```python
from build123d import *

# Parameters (mm, degrees)
ESQUISSE1_W             = 15
ESQUISSE1_H             = 11
BOSS_EXTRU_1_DEPTH      = 7.5
ESQUISSE2_R             = 1.5
ENL_V_MAT_EXTRU_1_DEPTH = 12.947803145
CONG_1_R                = 2
CONG_2_R                = 0.5


with BuildPart() as part:
    # Esquisse1 → Boss.-Extru.1 (new body)
    with BuildSketch(Plane.XY):
        Rectangle(ESQUISSE1_W, ESQUISSE1_H)
    extrude(amount=BOSS_EXTRU_1_DEPTH)

    # Esquisse2 → Enlèv. mat.-Extru.1 (cut, through all)
    with BuildSketch(Plane.XY.offset(7.5)):
        with Locations((0, 2)):
            Circle(ESQUISSE2_R)
    extrude(amount=-ENL_V_MAT_EXTRU_1_DEPTH, mode=Mode.SUBTRACT)

    # Congé1
    cong_1_edges = [part.edges().sort_by_distance(p)[0] for p in [
        (-7.5, 5.5, 3.75),
        (7.5, 5.5, 3.75),
    ]]
    fillet(cong_1_edges, radius=CONG_1_R)

    # Congé2
    cong_2_edges = [part.edges().sort_by_distance(p)[0] for p in [
        (7.5, -5.5, 3.75),
        (-7.5, -5.5, 3.75),
    ]]
    fillet(cong_2_edges, radius=CONG_2_R)


solid = part.part
```
Work out the finished part from the listing and answer in its coordinate system (mm). Give positions to 0.01 mm unless a question says otherwise; leave off trailing zeros. Write each loop counter-clockwise with the first axis right and the second up, starting at its lowest first coordinate (ties: lowest second). Pieces come first, ordered by that corner, then holes. Notation, with made-up numbers: (-24, 82) -> (10, 82) arc R24 cw to (10, 118) -> close; hole circle Ø5 at (65.25, 53). An arc over 180 degrees is marked (long way). Write item = value, one per line.
Q1. Section A-A on y = 2 is taken. Determine the outline of the cut face in (x, z).
Computed values:
outline = (-7.5, 0) -> (-1.5, 0) -> (-1.5, 7.5) -> (-7.5, 7.5) -> close; (1.5, 0) -> (7.5, 0) -> (7.5, 7.5) -> (1.5, 7.5) -> close
Q2. Consider line 1 along Y through (x, z) = (0, 3.25); line 2 along X through (y, z) = (2.5, 5); line 3 along X through (y, z) = (1.25, 4.75). Determine where each line is inside the solid, lowest interval first.
Computed values:
line_1 = -5.5 to 0.5, 3.5 to 5.5
line_2 = -7.5 to -1.41, 1.41 to 7.5
line_3 = -7.5 to -1.3, 1.3 to 7.5
Q3. Section B-B on x = 0 is taken. Determine the outline of the cut face in (y, z).
Computed values:
outline = (-5.5, 0) -> (0.5, 0) -> (0.5, 7.5) -> (-5.5, 7.5) -> close; (3.5, 0) -> (5.5, 0) -> (5.5, 7.5) -> (3.5, 7.5) -> close
Q4. Section C-C on z = 1.5 is taken. Determine the outline of the cut face in (x, y), and give its area (3 significant figures).
Computed values:
outline = (-7.5, -5) arc R0.5 ccw to (-7, -5.5) -> (7, -5.5) arc R0.5 ccw to (7.5, -5) -> (7.5, 3.5) arc R2 ccw to (5.5, 5.5) -> (-5.5, 5.5) arc R2 ccw to (-7.5, 3.5) -> close; hole circle Ø3 at (0, 2)
area = 156 mm^2
Q5. For a pull along Y with two mould halves and no side action, classify faces 1 (the flat face through (-7.5, -1, 4)), 2 (the cylindrical face through (-0.325, 0.536, 3.802)), 3 (the cylindrical face through (6.9, 4.93, 3.8)) as pulls with the +Y half, pulls with the -Y half, needs draft (parallel to the pull), parting line crosses it, or undercut.
Computed values:
face_1 = needs draft
face_2 = undercut
face_3 = pulls with the +Y half
